Can you work these out from the model? Positions are in its coordinate system, mm. A direction names the side the tool comes from. Coordinates: 2 decimals unless noted, no trailing zeros. Order: outer loops, then holes, each group sorted by start corner. A loop starts at its lowest first (then second) coordinate and runs counter-clockwise, first axis right, second up. Notation, with made-up numbers: (83, -2) -> (101, -2) arc R12 ccw to (101, 5) -> close; hole circle Ø4 at (22, 87). An arc over 180 degrees is marked (long way). Write item = value, one per line.
```python
from build123d import *

# Parameters (mm, degrees)
F0_W     = 22
F0_H     = 20
F1_DEPTH = 11.35
F2_R     = 1.075
F3_DEPTH = 22.001
F4_R     = 8.5
F5_DEPTH = 12.31


with BuildPart() as f1:
    # F0 (on Top) → F1 (new body)
    with BuildSketch(Plane.XY):
        Rectangle(F0_W, F0_H)
    extrude(amount=F1_DEPTH)

    # F2 (on face) → F3 (cut, through all)
    with BuildSketch(Plane(origin=(-11, 0, 0), x_dir=(0, -1, 0), z_dir=(-1, 0, 0))):
        with Locations((-6, 9.35)):
            Circle(F2_R)
        with Locations((0, 9.35)):
            Circle(F2_R)
        with Locations((6, 9.35)):
            Circle(F2_R)
    extrude(amount=-F3_DEPTH, mode=Mode.SUBTRACT)

    # F4 (on face) → F5 (join)
    with BuildSketch(Plane.XY.offset(11.35)):
        Circle(F4_R)
    extrude(amount=F5_DEPTH)


solid = f1.part
```
Item 1: I want a section at B-B, the plane z = 9.35. Please give me the cut outline in (x, y) (3 decimals).
A:
outline = (-11, -10) -> (11, -10) -> (11, -7.075) -> (-11, -7.075) -> close; (-11, -4.925) -> (11, -4.925) -> (11, -1.075) -> (-11, -1.075) -> close; (-11, 1.075) -> (11, 1.075) -> (11, 4.925) -> (-11, 4.925) -> close; (-11, 7.075) -> (11, 7.075) -> (11, 10) -> (-11, 10) -> close
Item 2: For faces 4 (the flat face through (-7.5, 4.6, 11.35)), 5 (the cylindrical face through (-0.2, 5.5, 8.4)), which set-ups out of +Z, -Z, +X, -X, +Y, -Y let a thin tool reach every point of the face, with its end or its side?
A:
face_4 = +Z
face_5 = +X, -X
Item 3: I'm going to push flat-ended pins straight in: P1, Ø4, axis at x = -8.5, z = 21, coming from the -Y side; P2, Ø3, axis at y = -4, z = 16, coming from the -X side; P3, Ø1.3, axis at y = 6, z = 9.35, coming from the -X side; P4, Ø8, axis at x = -4, z = 16.5, coming from the -Y side. Where does each tip first touch, or does it pass through?
A:
P1 = -5.48
P2 = -8.12
P3 = through
P4 = -8.5
Item 4: If I drill on probe 1 along Z at (x, y) = (-3.5, 6) (3 decimals); probe 2 along Y at (x, z) = (-1.75, 9.5); probe 3 along Z at (x, y) = (-8.5, 8), over which ranges is the centre line in solid material (lowest first)?
A:
probe_1 = 0 to 8.275, 10.425 to 23.66
probe_2 = -10 to -7.06, -4.94 to -1.06, 1.06 to 4.94, 7.06 to 10
probe_3 = 0 to 11.35
Item 5: If we mould it in two halves opening along Z, with no side actions, what happens to faces 1 (the flat face through (0, 0, 23.66)), 2 (the flat face through (-11, 0, 6)), 3 (the cylindrical face through (-0.15, 0.23, 8.3))? For each: pulls with the +Z half, pulls with the -Z half, needs draft (parallel to the pull), parting line crosses it, or undercut.
A:
face_1 = pulls with the +Z half
face_2 = needs draft
face_3 = undercut
Item 6: I want a section at A-A, the plane x = 0. Please give me the cut outline in (y, z) (3 decimals).
A:
outline = (-10, 0) -> (10, 0) -> (10, 11.35) -> (8.5, 11.35) -> (8.5, 23.66) -> (-8.5, 23.66) -> (-8.5, 11.35) -> (-10, 11.35) -> close; hole circle Ø2.15 at (-6, 9.35); hole circle Ø2.15 at (0, 9.35); hole circle Ø2.15 at (6, 9.35)
Item 7: I want a section at D-D, the plane y = 6. Please give me the cut outline in (x, z) (3 decimals), plus the area to 3 significant figures.
A:
outline = (-11, 0) -> (11, 0) -> (11, 8.275) -> (-11, 8.275) -> close; (-11, 10.425) -> (11, 10.425) -> (11, 11.35) -> (6.021, 11.35) -> (6.021, 23.66) -> (-6.021, 23.66) -> (-6.021, 11.35) -> (-11, 11.35) -> close
area = 351 mm2
Item 8: I want a section at C-C, the plane y = 0.75. Please give me the cut outline in (x, z).
A:
outline = (-11, 0) -> (11, 0) -> (11, 8.58) -> (-11, 8.58) -> close; (-11, 10.12) -> (11, 10.12) -> (11, 11.35) -> (8.47, 11.35) -> (8.47, 23.66) -> (-8.47, 23.66) -> (-8.47, 11.35) -> (-11, 11.35) -> close
